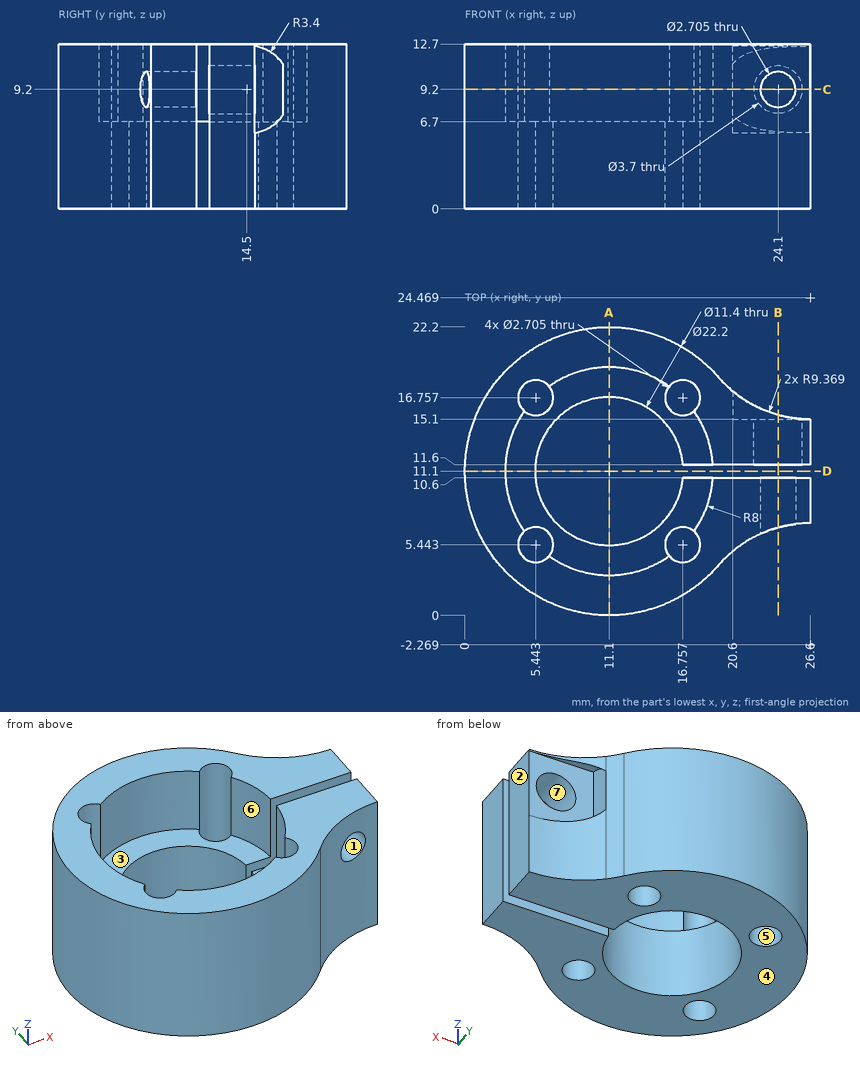
Could you check a few things on this drawing? It's one solid part, dimensions in mm from its lowest x, y, z. A direction names the side the tool comes from. Coordinates: 2 decimals unless noted, no trailing zeros. Order: outer loops, then holes, each group sorted by start corner. A loop starts at its lowest first (then second) coordinate and runs counter-clockwise, first axis right, second up.
1. If we section it at C-C (z = 9.2): Give the number of separate pieces and of enclosed holes in the cut face, then the cut area to 3 significant figures.
2. Thinking about a two-plate mould opening in Z: for the marked faces 1, 2, 3 and 4, which applies, +Z half, -Z half, draft (parallel to the pull), parting line (faces both ways), or undercut?
3. I need wall thicknesses on line 1 (Y direction, x = 11, z = 8); line 2 (Z direction, x = 24.1, y = 13); line 3 (Y direction, x = 17, z = 4). Which ranges of each line are inside material? Lowest first, please.
4. If we section it at A-A (x = 11.1): Please give me the cut outline in (y, z), then the cut area to 3 significant figures.
5. For the marked faces 5, 6 and 7, which set-ups out of +Z, -Z, +X, -X, +Y, -Y let a thin tool reach every point of the face, with its end or its side?
6. If we section it at B-B (x = 24.1): Please give me the cut outline in (y, z).
7. If we section it at D-D (y = 11.1): Please give me the cut outline in (x, z).
8. I'm going to push flat-ended pins straight in: pin 1 (4.5 mm diameter, centred on x = 5.44, y = 5.44, fed in from -Z); pin 2 (5 mm diameter, centred on y = 4, z = 2, fed in from -X); pin 3 (6 mm diameter, centred on x = 21.5, z = 2, fed in from -Y); pin 4 (4.5 mm diameter, centred on x = 24.1, z = 9.2, fed in from +Y). Where does each tip first touch, or does it pass through?
Entries:
1. separate pieces: 3
1. enclosed holes: 0
1. area: 183 mm2
2. face 1: undercut
2. face 2: draft
2. face 3: +Z half
2. face 4: -Z half
3. line 1: y = 0 to 3.1, 19.1 to 22.2
3. line 2: z = 0 to 7.35, 11.05 to 12.7
3. line 3: y = 1.7 to 4.11, 6.77 to 10.6, 11.6 to 15.43, 18.09 to 20.5
4. outline: (0, 0) - (5.4, 0) - (5.4, 6.7) - (3.1, 6.7) - (3.1, 12.7) - (0, 12.7) - close; (16.8, 0) - (22.2, 0) - (22.2, 12.7) - (19.1, 12.7) - (19.1, 6.7) - (16.8, 6.7) - close
4. area: 110 mm2
5. face 5: +Z, -Z
5. face 6: +Z
5. face 7: +Y
6. outline: (6.76, 0) - (10.6, 0) - (10.6, 7.85) - (6.76, 7.85) - close; (6.76, 10.55) - (10.6, 10.55) - (10.6, 12.7) - (6.76, 12.7) - close; (11.6, 0) - (15.44, 0) - (15.44, 5.93) arc R3.4 cw to (15.1, 5.85) - (15.1, 7.35) - (11.6, 7.35) - close; (11.6, 11.05) - (15.1, 11.05) - (15.1, 12.55) arc R3.4 cw to (15.44, 12.47) - (15.44, 12.7) - (11.6, 12.7) - close
7. outline: (0, 0) - (5.4, 0) - (5.4, 6.7) - (3.1, 6.7) - (3.1, 12.7) - (0, 12.7) - close
8. pin 1: stops at z = 0
8. pin 2: stops at x = 1
8. pin 3: stops at y = 2.83
8. pin 4: stops at y = 15.1
